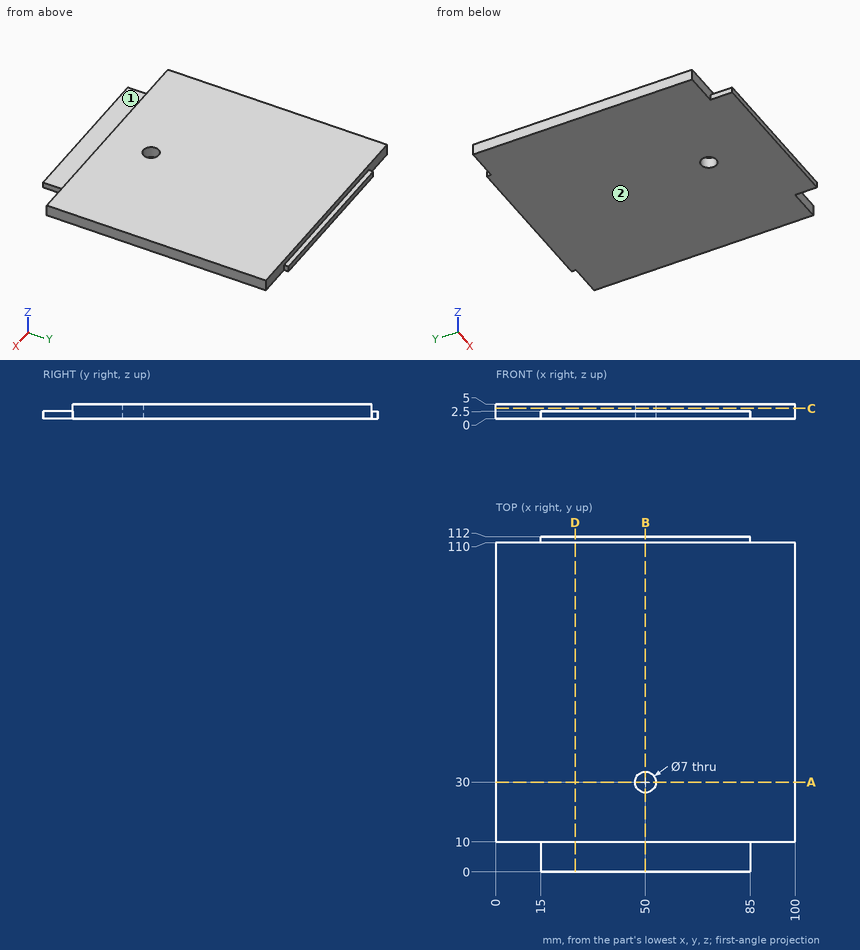
Check sheet for the drawn part. Datum: minimum x, y, z corner. Units: mm. A direction names the side the tool comes from. Give positions to 0.01 mm unless a question says otherwise; leave off trailing zeros. Order: outer loops, then holes, each group sorted by start corner. A loop starts at its lowest first (then second) coordinate and runs counter-clockwise, first axis right, second up. Notation, with made-up numbers: (-27, -20) -> (-15, -20) arc R17 cw to (-15, 4) -> close; hole circle Ø6 at (29, 40). An arc over 180 degrees is marked (long way). One line per item, written item: value.
(1) Sectioned sample at D-D on x = 26.5. Record the cut outline in (y, z), then the cut area to 3 significant figures.
Final values:
outline: (0, 0) -> (112, 0) -> (112, 2.5) -> (110, 2.5) -> (110, 5) -> (10, 5) -> (10, 2.5) -> (0, 2.5) -> close
area: 530 mm^2
(2) Gauge pin test, flat ends, axial feed: pin 1 (3 mm diameter, centred on y = 4, z = 1, fed in from -X); pin 2 (2 mm diameter, centred on y = 3.5, z = 1.5, fed in from +X); pin 3 (2 mm diameter, centred on x = 11.5, z = 4.5, fed in from -Y). Record the tip position at first contact, or that the pin passes through.
Final values:
pin 1: x = 15
pin 2: x = 85
pin 3: y = 10
(3) Tool access check on the marked faces 1 and 2. Record the directions out of +Z, -Z, +X, -X, +Y, -Y that give a thin tool (end or side, any length) a straight path to the whole face; none if there is none.
Final values:
face 1: +Z, +X, -X, -Y
face 2: -Z, +X, -X, +Y, -Y
(4) Sectioned sample at A-A on y = 30. Record the cut outline in (x, z).
Final values:
outline: (0, 0) -> (46.5, 0) -> (46.5, 5) -> (0, 5) -> close; (53.5, 0) -> (100, 0) -> (100, 5) -> (53.5, 5) -> close
(5) Sectioned sample at C-C on z = 3.55. Record the cut outline in (x, y).
Final values:
outline: (0, 10) -> (100, 10) -> (100, 110) -> (0, 110) -> close; hole circle Ø7 at (50, 30)
(6) Sectioned sample at B-B on x = 50. Record the cut outline in (y, z), then the cut area to 3 significant figures.
Final values:
outline: (0, 0) -> (26.5, 0) -> (26.5, 5) -> (10, 5) -> (10, 2.5) -> (0, 2.5) -> close; (33.5, 0) -> (112, 0) -> (112, 2.5) -> (110, 2.5) -> (110, 5) -> (33.5, 5) -> close
area: 495 mm^2
(7) Scan lines: line 1 along X through (y, z) = (30, 3.9); line 2 along Y through (x, z) = (50, 2.75); line 3 along Y through (x, z) = (35, 4.8). Record each from-to range of solid material in increasing order. Write a range as [from, to].
Final values:
line 1: [0, 46.5], [53.5, 100]
line 2: [10, 26.5], [33.5, 110]
line 3: [10, 110]
